For this review, take the finished solid that the model builds, in its own axes (mm). Coordinates: 2 decimals unless noted, no trailing zeros. Loops run counter-clockwise (first coordinate to the right, second up) from the corner with the lowest first, then second, coordinate; pieces in that order, holes last. Notation, with made-up numbers: (59.5, 66.5) - (78.5, 66.5) arc R9 cw to (78.5, 71.5) - close; hole circle Ø10 at (66, 63). An arc over 180 degrees is marked (long way). One line per item, written item: value. Start each with the question number.
1. Take a section at A-A, the plane x = 0. State the section outline as (y, z) points.
2. Take a section at C-C, the plane y = 40. State the section outline as (x, z) points.
3. Take a section at B-B, the plane x = 42.5. State the section outline as (y, z) points.
4. Take a section at D-D, the plane z = 1.2. Count the separate pieces of the cut face and the enclosed holes in it, and give its area (3 significant figures).
5. To check wall thickness, follow line 1 (Y direction, x = 0, z = 0.9); line 2 (X direction, y = 26, z = 2.55); line 3 (X direction, y = 13, z = 2.8). State the ranges of each line that lie inside material, in increasing order. Write a range as from..to.
6. Insertion check: pin 1 (3 mm diameter, centred on x = -25, y = 0, fed in from +Z); pin 2 (1 mm diameter, centred on y = 13, z = 1, fed in from +X). Each pin has a flat end and moves straight along its axis. Give the tip position at first contact, or say it passes through.
```python
from build123d import *

# Parameters (mm, degrees)
SKETCH2_R           = 2.5
BOSS_EXTRUDE1_DEPTH = 3


with BuildPart() as part:
    # Sketch2 → Boss-Extrude1 (new body)
    with BuildSketch(Plane.XY):
        with BuildLine():
            Line((-61.770239404, 32.654595977), (-5.310718211, 54.028409464))
            ThreePointArc((-5.310718211, 54.028409464), (0, 55), (5.310718211, 54.028409464))
            Line((5.310718211, 54.028409464), (61.770239404, 32.654595977))
            ThreePointArc((61.770239404, 32.654595977), (64.939100687, 28.75645975), (63.122009394, 24.072943218))
            Line((63.122009394, 24.072943218), (28.122009394, -3.905516271))
            ThreePointArc((28.122009394, -3.905516271), (26.654149123, -4.718452149), (25, -5))
            Line((25, -5), (0, -5))
            Line((0, -5), (-25, -5))
            ThreePointArc((-25, -5), (-26.654149123, -4.718452149), (-28.122009394, -3.905516271))
            Line((-28.122009394, -3.905516271), (-63.122009394, 24.072943218))
            ThreePointArc((-63.122009394, 24.072943218), (-64.939100687, 28.75645975), (-61.770239404, 32.654595977))
        make_face()
        with Locations((-60, 27.978459489)):
            Circle(SKETCH2_R, mode=Mode.SUBTRACT)
        with Locations((0, 40)):
            Circle(SKETCH2_R, mode=Mode.SUBTRACT)
        with Locations((60, 27.978459489)):
            Circle(SKETCH2_R, mode=Mode.SUBTRACT)
        with Locations((25, 0)):
            Circle(SKETCH2_R, mode=Mode.SUBTRACT)
        Circle(SKETCH2_R, mode=Mode.SUBTRACT)
        with Locations((-25, 0)):
            Circle(SKETCH2_R, mode=Mode.SUBTRACT)
        with Locations((-42.5, 13.989229745)):
            Circle(SKETCH2_R, mode=Mode.SUBTRACT)
        with Locations((42.5, 13.989229745)):
            Circle(SKETCH2_R, mode=Mode.SUBTRACT)
    extrude(amount=BOSS_EXTRUDE1_DEPTH)


solid = part.part
```
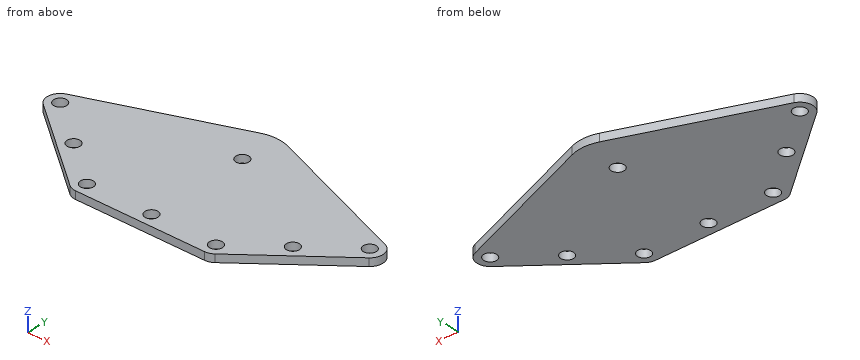
Solutions:
1. outline: (-5, 0) - (-2.5, 0) - (-2.5, 3) - (-5, 3) - close; (2.5, 0) - (37.5, 0) - (37.5, 3) - (2.5, 3) - close; (42.5, 0) - (55, 0) - (55, 3) - (42.5, 3) - close
2. outline: (-42.37, 0) - (-2.5, 0) - (-2.5, 3) - (-42.37, 3) - close; (2.5, 0) - (42.37, 0) - (42.37, 3) - (2.5, 3) - close
3. outline: (7.59, 0) - (11.49, 0) - (11.49, 3) - (7.59, 3) - close; (16.49, 0) - (39.95, 0) - (39.95, 3) - (16.49, 3) - close
4. separate pieces: 1
4. enclosed holes: 8
4. area: 5,000 mm2
5. line 1: -5..-2.5, 2.5..37.5, 42.5..55
5. line 2: -64.59..-61.53, -58.47..58.47, 61.53..64.59
5. line 3: -49.27..-44.8, -40.2..40.2, 44.8..49.27
6. pin 1: through
6. pin 2: x = 49.9
